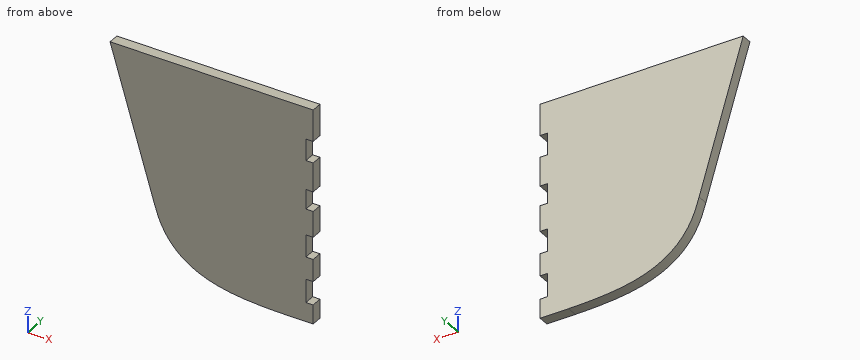
from build123d import *

# Parameters (mm, degrees)
BOSS_EXTRUDE1_DEPTH = 5.715


with BuildPart() as part:
    # Sketch1 → Boss-Extrude1 (new body)
    with BuildSketch(Plane(origin=(0, 0, 0), x_dir=(1, 0, 0), z_dir=(0, 1, 0))):
        with BuildLine():
            Line((23.434979066, 78.109868229), (0, 0))
            Line((0, 0), (107.95, 0))
            Line((107.95, 0), (107.95, 16.763624127))
            Line((107.95, 16.763624127), (104.075854958, 16.763624127))
            Line((104.075854958, 16.763624127), (104.075854958, 28.274535242))
            Line((104.075854958, 28.274535242), (107.95, 28.274535242))
            Line((107.95, 28.274535242), (107.95, 43.736953157))
            Line((107.95, 43.736953157), (104.075854958, 43.736953157))
            Line((104.075854958, 43.736953157), (104.075854958, 54.217036411))
            Line((104.075854958, 54.217036411), (107.95, 54.217036411))
            Line((107.95, 54.217036411), (107.95, 67.961407891))
            Line((107.95, 67.961407891), (104.075854958, 67.961407891))
            Line((104.075854958, 67.961407891), (104.075854958, 79.815928293))
            Line((104.075854958, 79.815928293), (107.95, 79.815928293))
            Line((107.95, 79.815928293), (107.95, 91.670448695))
            Line((107.95, 91.670448695), (104.075854958, 91.670448695))
            Line((104.075854958, 91.670448695), (104.075854958, 104.11377721))
            Line((104.075854958, 104.11377721), (107.95, 104.11377721))
            Line((107.95, 104.11377721), (107.95, 114.3))
            Line((107.95, 114.3), (92.782636258, 114.3))
            add(Edge.make_bspline(
                [(23.434979066, 78.109868229), (23.977674271, 79.918696425), (33.365084494, 111.207368521), (62.592771748, 114.091936467), (92.782636258, 114.3)],
                knots=[0, 0, 0, 0, 0.05, 0.864887892, 0.864887892, 0.864887892, 0.864887892], degree=3))
        make_face()
    extrude(amount=BOSS_EXTRUDE1_DEPTH)


solid = part.part
Work out the finished part from the listing and answer in its coordinate system (mm). Give positions to 0.01 mm unless a question says otherwise; leave off trailing zeros. Loops run counter-clockwise (first coordinate to the right, second up) from the corner with the lowest first, then second, coordinate; pieces in that order, holes last. Notation, with made-up numbers: (-15, 64) - (31, 64) arc R9 ccw to (31, 74) - close; hole circle Ø3 at (49, 68.25). An arc over 180 degrees is marked (long way). Answer in a Markdown table with one row per item. Add a question column.
Q1. Consider line 1 along Z through (x, y) = (92, 5.15); line 2 along X through (y, z) = (3.9, -80.5); line 3 along Z through (x, y) = (28, 3.45). Determine where each line is inside the solid, lowest interval first.
Q2. The part is cut by section A-A (z = -38.5). Determine the outline of the cut face in (x, y) (3 decimals).
Q3. The part is cut by section B-B (x = 14.5). Determine the outline of the cut face in (y, z) (3 decimals).
Q4. Each of these flat-tipped pins is pushed along its axis until it touches: P1, Ø3, axis at x = 19, y = 3.5, coming from the +Z side; P2, Ø3, axis at y = 2.5, z = -75.5, coming from the +X side; P3, Ø2, axis at x = 72, y = 4.5, coming from the -Z side. Where does it stop, or does it pass through?
Solution:
| question | item | result |
|---|---|---|
| 1 | line 1 | z = -114.29 to 0 |
| 1 | line 2 | x = 24.16 to 107.95 |
| 1 | line 3 | z = -89.97 to 0 |
| 2 | outline | (11.551, 0) - (107.95, 0) - (107.95, 5.715) - (11.551, 5.715) - close |
| 3 | outline | (0, -48.329) - (5.715, -48.329) - (5.715, 0) - (0, 0) - close |
| 4 | P1 | stops at z = 0 |
| 4 | P2 | stops at x = 104.08 |
| 4 | P3 | stops at z = -113.52 |
